Check sheet for the modelled part. Datum: model origin and axes. Units: mm. A direction names the side the tool comes from. Round coordinates to 2 decimals unless told otherwise and drop trailing zeros. Order: outer loops, then holes, each group sorted by start corner. A loop starts at its lowest first (then second) coordinate and runs counter-clockwise, first axis right, second up. Notation, with made-up numbers: (55, -32) -> (71, -32) arc R37 ccw to (71, 6) -> close; hole circle Ø10 at (-14, -19). An arc over 180 degrees is marked (long way). Answer in a Markdown table with one row per item.
from build123d import *

# Parameters (mm, degrees)
F0_W     = 101.6
F0_H     = 63.5
F1_DEPTH = 25.4
F2_DEPTH = 50.8
F4_R     = 51.3264150983
F5_DEPTH = 117.602
F6_W     = 50.8
F6_H     = 12.3184835084
F7_DEPTH = 25.4
F8_DEPTH = 25.4


with BuildPart() as f1:
    # F0 (on Top) → F1 (new body)
    with BuildSketch(Plane.XY):
        with Locations((47.4951000333, -21.5426209271)):
            Rectangle(F0_W, F0_H)
    extrude(amount=F1_DEPTH)

    # F2 (add): a face of the model
    f2_faces = [f1.faces().sort_by_distance(p)[0] for p in [
        (47.4951000333, -21.5426209271, 25.4),
    ]]
    extrude(f2_faces, amount=F2_DEPTH)

    # F4 (on face) → F5 (cut)
    with BuildSketch(Plane.YZ.offset(98.2951000333)):
        with Locations((-53.4369722009, 76.4370337129)):
            Circle(F4_R)
    extrude(amount=-F5_DEPTH, mode=Mode.SUBTRACT)

    # F6 (on face) → F7 (cut)
    with BuildSketch(Plane.XY.offset(76.2)):
        with Locations((47.4951000333, 4.0481373187)):
            Rectangle(F6_W, F6_H)
    extrude(amount=-F7_DEPTH, mode=Mode.SUBTRACT)

    # F8 (cut): a face of the model
    f8_faces = [f1.faces().sort_by_distance(p)[0] for p in [
        (47.4951000333, -2.1111044355, 63.5),
    ]]
    extrude(f8_faces, amount=-F8_DEPTH, mode=Mode.SUBTRACT)


solid = f1.part
Item 1: Set-up check for faces 4 (the flat face through (9, 4, 76.2)), 5 (the flat face through (47, 1, 50.8)): record each of +Z, -Z, +X, -X, +Y, -Y from which the full face is reachable in a straight line by a thin tool's end or side.
Result sheet:
| item | result |
|---|---|
| face 4 | +Z, +X, -X, +Y, -Y |
| face 5 | +Z, +Y, -Y |
Item 2: Scan lines: line 1 (Z direction, x = 30, y = 6.5); line 2 (Z direction, x = 72.5, y = -13.5); line 3 (Y direction, x = 35, z = 45). Record each from-to range of solid material in increasing order. Write a range as [from, to].
Result sheet:
| item | result |
|---|---|
| line 1 | z = [0, 50.8] |
| line 2 | z = [0, 44.2] |
| line 3 | y = [-12.86, 10.21] |
Item 3: Mould release check, pull along X, two halves, no side actions. Record for faces 1 (the flat face through (22.095, 3, 64)), 2 (the flat face through (98.295, -15, 29)), 3 (the flat face through (47, -53.293, 12)): pulls with the +X half, pulls with the -X half, needs draft (parallel to the pull), parting line crosses it, or undercut.
Result sheet:
| item | result |
|---|---|
| face 1 | undercut |
| face 2 | pulls with the +X half |
| face 3 | needs draft |
Item 4: Cross-section at B-B (y = 1.5). Record the boundary of the cut face in (x, z).
Result sheet:
| item | result |
|---|---|
| outline | (-3.3, 0) -> (98.3, 0) -> (98.3, 76.2) -> (72.9, 76.2) -> (72.9, 50.8) -> (22.1, 50.8) -> (22.1, 76.2) -> (-3.3, 76.2) -> close |
Item 5: Depth check by flat-ended pin: P1, Ø5, axis at y = -31.5, z = 34.5, coming from the +X side; P2, Ø15.5, axis at x = 41, y = 3.5, coming from the +Z side. Enter the tip coordinate at first touch or a pass-through.
Result sheet:
| item | result |
|---|---|
| P1 | passes through |
| P2 | stops at z = 50.8 |
Item 6: Cross-section at D-D (z = 34). Record the boundary of the cut face in (x, y).
Result sheet:
| item | result |
|---|---|
| outline | (-3.3, -24.57) -> (98.3, -24.57) -> (98.3, 10.21) -> (-3.3, 10.21) -> close |
Item 7: Cross-section at A-A (z = 71). Record the boundary of the cut face in (x, y), and give its area (3 significant figures).
Result sheet:
| item | result |
|---|---|
| outline | (-3.3, -2.4) -> (22.1, -2.4) -> (22.1, 10.21) -> (-3.3, 10.21) -> close; (72.9, -2.4) -> (98.3, -2.4) -> (98.3, 10.21) -> (72.9, 10.21) -> close |
| area | 640 mm^2 |
Item 8: Cross-section at C-C (x = 89). Record the boundary of the cut face in (y, z).
Result sheet:
| item | result |
|---|---|
| outline | (-53.29, 0) -> (10.21, 0) -> (10.21, 76.2) -> (-2.11, 76.2) arc R51.33 cw to (-53.29, 25.11) -> close |
